from build123d import *

# Parameters (mm, degrees)
SKETCH1_R           = 10.5
BOSS_EXTRUDE1_DEPTH = 2.5
SKETCH2_R           = 3.5
SKETCH2_R_2         = 2.5
BOSS_EXTRUDE2_DEPTH = 3
SKETCH3_R           = 1.5
CUT_EXTRUDE1_DEPTH  = 3
CUT_EXTRUDE2_START  = -1.5
SKETCH4_R           = 4.5
SKETCH4_R_2         = 1.5
CUT_EXTRUDE2_DEPTH  = 1.5
SKETCH5_R           = 1
CUT_EXTRUDE3_DEPTH  = 3


with BuildPart() as part:
    # Sketch1 → Boss-Extrude1 (new body)
    with BuildSketch(Plane(origin=(0, 0, 0), x_dir=(1, 0, 0), z_dir=(0, 1, 0))):
        with Locations(Location((0, 0, 0), (0, 0, 270))):
            Circle(SKETCH1_R)
    extrude(amount=BOSS_EXTRUDE1_DEPTH)

    # Sketch2 → Boss-Extrude2 (add)
    with BuildSketch(Plane(origin=(0, 2.5, 0), x_dir=(1, 0, 0), z_dir=(0, 1, 0))):
        with Locations(Location((0, 0, 0), (0, 0, 270))):
            Circle(SKETCH2_R)
        with Locations(Location((0, 0, 0), (0, 0, 270))):
            Circle(SKETCH2_R_2, mode=Mode.SUBTRACT)
    extrude(amount=BOSS_EXTRUDE2_DEPTH)

    # Sketch3 → Cut-Extrude1 (cut)
    with BuildSketch(Plane(origin=(0, 2.5, 0), x_dir=(1, 0, 0), z_dir=(0, 1, 0))):
        with Locations(Location((0, 0, 0), (0, 0, 270))):
            Circle(SKETCH3_R)
    extrude(amount=-CUT_EXTRUDE1_DEPTH, mode=Mode.SUBTRACT)

    # Sketch4 → Cut-Extrude2 (cut)
    with BuildSketch(Plane.XZ.offset(CUT_EXTRUDE2_START)):
        with Locations(Location((0, 0, 0), (0, 0, 270))):
            Circle(SKETCH4_R)
        with Locations(Location((0, 0, 0), (0, 0, 90))):
            Circle(SKETCH4_R_2, mode=Mode.SUBTRACT)
    extrude(amount=CUT_EXTRUDE2_DEPTH, mode=Mode.SUBTRACT)

    # Sketch5 → Cut-Extrude3 (cut)
    with BuildSketch(Plane.XZ):
        with Locations(Location((0, 7, 0), (0, 0, 270))):
            Circle(SKETCH5_R)
        with Locations(Location((3.5, 7, 0), (0, 0, 270))):
            Circle(SKETCH5_R)
        with Locations(Location((-3.5, 7, 0), (0, 0, 270))):
            Circle(SKETCH5_R)
        with Locations(Location((7, 3.5, 0), (0, 0, 270))):
            Circle(SKETCH5_R)
        with Locations(Location((7, 0, 0), (0, 0, 270))):
            Circle(SKETCH5_R)
        with Locations(Location((7, -3.5, 0), (0, 0, 270))):
            Circle(SKETCH5_R)
        with Locations(Location((3.5, -7, 0), (0, 0, 270))):
            Circle(SKETCH5_R)
        with Locations(Location((0, -7, 0), (0, 0, 270))):
            Circle(SKETCH5_R)
        with Locations(Location((-3.5, -7, 0), (0, 0, 270))):
            Circle(SKETCH5_R)
        with Locations(Location((-7, -3.5, 0), (0, 0, 270))):
            Circle(SKETCH5_R)
        with Locations(Location((-7, 0, 0), (0, 0, 270))):
            Circle(SKETCH5_R)
        with Locations(Location((-7, 3.5, 0), (0, 0, 270))):
            Circle(SKETCH5_R)
    extrude(amount=-CUT_EXTRUDE3_DEPTH, mode=Mode.SUBTRACT)


solid = part.part
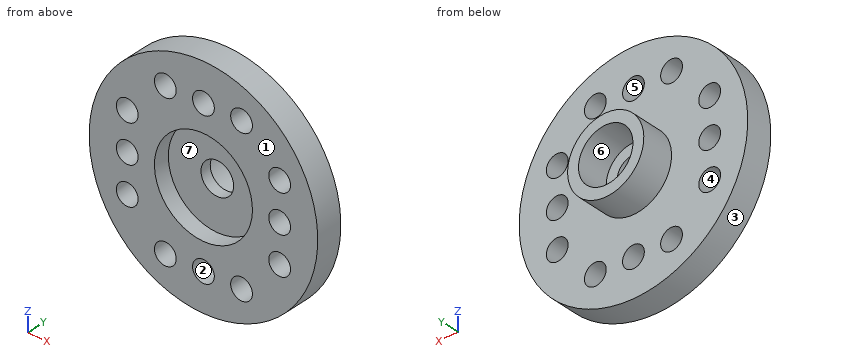
Read the model definition and answer for the solid it produces. Units are mm, in the model's axes. Face numbers are marked on the shaded views. A direction names the side the tool comes from. Give positions to 0.01 mm unless a question says otherwise; leave off trailing zeros. Write each loop counter-clockwise with the first axis right and the second up, starting at its lowest first coordinate (ties: lowest second). Pieces come first, ordered by that corner, then holes. Notation, with made-up numbers: (49, -29.75) -> (80, -29.75) arc R8 cw to (80, -25.75) -> close; hole circle Ø6 at (56.5, 65). An arc over 180 degrees is marked (long way). Answer as a JSON object with one key per item and string values. Group by question number.
1) Find section D-D (x = 3). Write down the section's boundary in (y, z).
2) Consider L1, parallel to X at y = 2.2, z = 0; L2, parallel to X at y = 0.7, z = 0; L3, parallel to X at y = 2.3, z = 3.25. Determine where each line is inside the solid, lowest interval first. Write a range as from..to.
3) Find section B-B (x = -7.75). Write down the section's boundary in (y, z), and give its area (3 significant figures).
4) Find section C-C (z = -7). Write down the section's boundary in (x, y), and give its area (3 significant figures).
5) A tool of negligible diameter and unlimited length cuts with its end or side. For the marked faces 5, 6 and 7, from which of +Z, -Z, +X, -X, +Y, -Y can it reach the whole face along a straight path? Write none if from no direction.
6) Find section A-A (y = 0.45). Count the separate pieces of the cut face and the enclosed holes in it, and give its area (3 significant figures).
7) The mould has two halves that part along X. Classify the marked faces 1, 2, 3 and 4: +X half, -X half, draft (parallel to the pull), parting line (faces both ways), or undercut.
8) Each of these flat-tipped pins is pushed along its axis until it touches: P1, Ø2.5, axis at x = 0, z = 7, coming from the +Y side; P2, Ø1, axis at y = 1.5, z = -6.5, coming from the +X side. Where does it stop, or does it pass through?
Values follow:
{
 "1": {"outline": "(0, -10.06) -> (2.5, -10.06) -> (2.5, -7.87) -> (0, -7.87) -> close; (0, -6.13) -> (2.5, -6.13) -> (2.5, -1.8) -> (5.5, -1.8) -> (5.5, 1.8) -> (2.5, 1.8) -> (2.5, 6.13) -> (0, 6.13) -> (0, 3.35) -> (1.5, 3.35) -> (1.5, -3.35) -> (0, -3.35) -> close; (0, 7.87) -> (2.5, 7.87) -> (2.5, 10.06) -> (0, 10.06) -> close"},
 "2": {"L1": "x = -10.5..-8, -6..-1.5, 1.5..6, 8..10.5", "L2": "x = -10.5..-8, -6..-4.5, 4.5..6, 8..10.5", "L3": "x = -9.98..-7.97, -6.03..6.03, 7.97..9.98"},
 "3": {"outline": "(0, -7.08) -> (2.5, -7.08) -> (2.5, -4.16) -> (0, -4.16) -> close; (0, -2.84) -> (2.5, -2.84) -> (2.5, -0.66) -> (0, -0.66) -> close; (0, 0.66) -> (2.5, 0.66) -> (2.5, 2.84) -> (0, 2.84) -> close; (0, 4.16) -> (2.5, 4.16) -> (2.5, 7.08) -> (0, 7.08) -> close", "area": "25.5 mm2"},
 "4": {"outline": "(-7.83, 0) -> (-4.5, 0) -> (-4.5, 2.5) -> (-7.83, 2.5) -> close; (-2.5, 0) -> (-1, 0) -> (-1, 2.5) -> (-2.5, 2.5) -> close; (1, 0) -> (2.5, 0) -> (2.5, 2.5) -> (1, 2.5) -> close; (4.5, 0) -> (7.83, 0) -> (7.83, 2.5) -> (4.5, 2.5) -> close", "area": "24.1 mm2"},
 "5": {"face 5": "+Y, -Y", "face 6": "+Y", "face 7": "-Y"},
 "6": {"separate pieces": "1", "enclosed holes": "13", "area": "245 mm2"},
 "7": {"face 1": "draft", "face 2": "undercut", "face 3": "parting line", "face 4": "undercut"},
 "8": {"P1": "stops at y = 2.5", "P2": "stops at x = 8.62"}
}
